from build123d import *

# Parameters (mm, degrees)
SKETCH1_W           = 210
SKETCH1_H           = 270
SKETCH1_R           = 7.75
BOSS_EXTRUDE2_DEPTH = 6
CUT_EXTRUDE1_DEPTH  = 10
SKETCH4_R           = 1.25
CUT_EXTRUDE2_DEPTH  = 10


with BuildPart() as part:
    # Sketch1 → Boss-Extrude2 (new body)
    with BuildSketch(Plane(origin=(0, 0, 0), x_dir=(1, 0, 0), z_dir=(0, 1, 0))):
        with Locations((0, -10)):
            Rectangle(SKETCH1_W, SKETCH1_H)
        with Locations(Location((0, 0, 0), (0, 0, 270))):
            Circle(SKETCH1_R, mode=Mode.SUBTRACT)
    extrude(amount=BOSS_EXTRUDE2_DEPTH)

    # Sketch3 → Cut-Extrude1 (cut)
    with BuildSketch(Plane.XZ):
        with BuildLine():
            Line((17.000022153, 29.5), (17.000022153, 9.5))
            ThreePointArc((17.000022153, 9.5), (15.500022153, 8), (14.000022153, 9.5))
            Line((14.000022153, 9.5), (14.000022153, 29.5))
            ThreePointArc((14.000022153, 29.5), (15.500022153, 31), (17.000022153, 29.5))
        make_face()
        with BuildLine():
            Line((17.000022153, 60.5), (17.000022153, 40.5))
            ThreePointArc((17.000022153, 40.5), (15.500022153, 39), (14.000022153, 40.5))
            Line((14.000022153, 40.5), (14.000022153, 60.5))
            ThreePointArc((14.000022153, 60.5), (15.500022153, 62), (17.000022153, 60.5))
        make_face()
        with BuildLine():
            Line((-16.999993108, 29.500016738), (-17.0000128, 9.500016738))
            ThreePointArc((-17.0000128, 9.500016738), (-15.500014277, 8.000015261), (-14.0000128, 9.500013784))
            Line((-14.0000128, 9.500013784), (-13.999993108, 29.500013784))
            ThreePointArc((-13.999993108, 29.500013784), (-15.499991631, 31.000015261), (-16.999993108, 29.500016738))
        make_face()
        with BuildLine():
            Line((-16.999962586, 60.500016738), (-16.999982277, 40.500016738))
            ThreePointArc((-16.999982277, 40.500016738), (-15.499983754, 39.000015261), (-13.999982277, 40.500013784))
            Line((-13.999982277, 40.500013784), (-13.999962586, 60.500013784))
            ThreePointArc((-13.999962586, 60.500013784), (-15.499961109, 62.000015261), (-16.999962586, 60.500016738))
        make_face()
        with BuildLine():
            Line((11.250022153, 44.999994462), (11.250012307, 24.999994462))
            ThreePointArc((11.250012307, 24.999994462), (6.769e-06, 13.75), (-11.249987693, 25.000005538))
            Line((-11.249987693, 25.000005538), (-11.249977847, 45.000005538))
            ThreePointArc((-11.249977847, 45.000005538), (2.7692e-05, 56.25), (11.250022153, 44.999994462))
        make_face()
    extrude(amount=-CUT_EXTRUDE1_DEPTH, mode=Mode.SUBTRACT)

    # Sketch4 → Cut-Extrude2 (cut)
    with BuildSketch(Plane.XZ):
        with Locations(Location((49.170333674, -115.382230576, 0), (0, 0, 270))):
            Circle(SKETCH4_R)
        with Locations(Location((-44.829666326, -115.382230576, 0), (0, 0, 270))):
            Circle(SKETCH4_R)
        with Locations(Location((49.170333674, -40.382230576, 0), (0, 0, 270))):
            Circle(SKETCH4_R)
        with Locations(Location((-44.829666326, -40.382230576, 0), (0, 0, 270))):
            Circle(SKETCH4_R)
    extrude(amount=-CUT_EXTRUDE2_DEPTH, mode=Mode.SUBTRACT)


solid = part.part
Geometry: final body of the model. Coordinates: model frame, mm. A direction names the side the tool comes from. Round coordinates to 2 decimals unless told otherwise and drop trailing zeros. Order: outer loops, then holes, each group sorted by start corner. A loop starts at its lowest first (then second) coordinate and runs counter-clockwise, first axis right, second up.
Q1. Section A-A, the plane z = 0. Output: boundary loops of the cut face in (x, y).
Result sheet:
outline: (-105, 0) - (-7.75, 0) - (-7.75, 6) - (-105, 6) - close; (7.75, 0) - (105, 0) - (105, 6) - (7.75, 6) - close
Q2. Mould query, pull axis Z, two halves, no side actions, for faces 1 (the face through (-1, 0, 8)), 2 (the face through (-11.25, 3, 35)), 3 (the face through (-1, 3, -125)). Classes: released by +Z, released by -Z, zero draft, split by the parting line, or undercut.
Result sheet:
face 1: zero draft
face 2: undercut
face 3: released by -Z
Q3. Section B-B, the plane y = 1. Give the number of separate pieces and of enclosed holes in the cut face, and give its area (3 significant figures).
Result sheet:
separate pieces: 1
enclosed holes: 10
area: 55,400 mm2
Q4. Material intervals for probe 1 along Z at (x, y) = (-45, 5); probe 2 along Z at (x, y) = (-15.5, 3); probe 3 along X at (y, z) = (1.75, 29), sorted ascending.
Result sheet:
probe 1: z = -125 to -116.62, -114.14 to -41.62, -39.14 to 145
probe 2: z = -125 to 8, 31 to 39, 62 to 145
probe 3: x = -105 to -17, -14 to -11.25, 11.25 to 14, 17 to 105
Q5. Access query for faces 4 (the face through (-1, 3, 145)), 5 (the face through (0.247, 2.958, 13.753)). Directions: +Z, -Z, +X, -X, +Y, -Y. A direction counts if a zero-diameter tool reaches every point of the face in a straight line with its end or side. Return the directions, or none.
Result sheet:
face 4: +Z, +X, -X, +Y, -Y
face 5: +Y, -Y
